Check sheet for the modelled part. Datum: model origin and axes. Units: mm. Give positions to 0.01 mm unless a question says otherwise; leave off trailing zeros. Write each loop counter-clockwise with the first axis right and the second up, starting at its lowest first coordinate (ties: lowest second). Pieces come first, ordered by that corner, then holes. Notation, with made-up numbers: M 18.5,55.5 L 29.5,55.5 A26 ccw 29.5,73.5 Z; hole C -8.75,37 d8. An arc over 180 degrees is marked long. Use CSV: the item, a comma, the result in double quotes. Start each with the question number.
1. Mould release check, pull along X, two halves, no side actions. Record for faces 1 (the face through (76.833, 5.164, 1.252)), 2 (the face through (6.67, 11.11, 1.25)), 3 (the face through (39, 5, 2.54)): +X half, -X half, draft (parallel to the pull), parting line (faces both ways), or undercut.
2. Cross-section at C-C, the plane y = 8.75. Enter the section's corners in (x, z).
3. Cross-section at B-B, the plane z = 0.9. Enter the section's corners in (x, y) (3 decimals).
4. Cross-section at A-A, the plane y = 5.08. Enter the section's corners in (x, z) (3 decimals), and give its area (3 significant figures).
5. Cross-section at D-D, the plane y = 2. Enter the section's corners in (x, z).
6. Scan lines: line 1 (X direction, y = 5, z = 1.7); line 2 (Y direction, x = 74.93, z = 0.6) (3 decimals); line 3 (X direction, y = 6.75, z = 0.4). Record each from-to range of solid material in increasing order.
from build123d import *

# Parameters (mm, degrees)
SKETCH1_R           = 1.905
BOSS_EXTRUDE1_DEPTH = 2.54
FILLET7_R           = 5.08


with BuildPart() as part:
    # Sketch1 → Boss-Extrude1 (new body)
    with BuildSketch(Plane.XY):
        Polygon((5.08, 10.16), (6.35, 11.43), (40.005, 11.43), (40.005, -1.27), (6.35, -1.27), (5.08, 0), (0, 0), (0, 10.16), align=None)
        with Locations((5.08, 5.08)):
            Circle(SKETCH1_R, mode=Mode.SUBTRACT)
    extrude(amount=BOSS_EXTRUDE1_DEPTH)

    # Fillet7
    # the kernel refuses this fillet: 5.08 mm, written as the material it takes off along each edge
    with BuildSketch(Plane(origin=(6.35, -1.27, -5.225260413), x_dir=(1, 0, 0), z_dir=(0, 0, 1))) as fillet7_piece_1:
        with BuildLine():
            CenterArc((2.090104165, 5.08), FILLET7_R, 228.590377891, 41.409622109)
            Line((-1.27, 1.27), (-1.337202083, 1.1938))
            ThreePointArc((-1.337202083, 1.1938), (-0.706842049, 0.563157951), (-0.071842049, -0.071842049))
            Line((-0.071842049, -0.071842049), (0, -0.1016))
            Line((0, -0.1016), (2.090104165, -0.1016))
            Line((2.090104165, -0.1016), (2.090104165, 0))
        make_face()
    extrude(amount=12.990520825, mode=Mode.SUBTRACT)
    with BuildSketch(Plane(origin=(6.35, 11.43, -5.225260413), x_dir=(-0.7071067811865464, -0.7071067811865488, 0), z_dir=(0, 0, 1))) as fillet7_piece_2:
        with BuildLine():
            CenterArc((2.11417562, 5.070029277), FILLET7_R, 225, 41.409622109)
            Line((-1.477926828, 1.477926828), (-1.549768877, 1.40608478))
            Line((-1.549768877, 1.40608478), (-0.071842049, -0.071842049))
            Line((-0.071842049, -0.071842049), (0, -0.1016))
            ThreePointArc((0, -0.1016), (0.898025612, -0.1016), (1.789688736, -0.101400586))
            Line((1.789688736, -0.101400586), (1.796051224, 0))
        make_face()
    extrude(amount=12.990520825, mode=Mode.SUBTRACT)
    with BuildSketch(Plane(origin=(0, 0, -12.7), x_dir=(1, 0, 0), z_dir=(0, 0, 1)), Plane(origin=(0, 10.16, -12.7), x_dir=(0, -1, 0), z_dir=(0, 0, 1))) as fillet7_piece_3:
        with BuildLine():
            CenterArc((FILLET7_R, FILLET7_R), FILLET7_R, 180, 90)
            Line((0, FILLET7_R), (-FILLET7_R * 0.02, FILLET7_R))
            Line((-FILLET7_R * 0.02, FILLET7_R), (-FILLET7_R * 0.02, -FILLET7_R * 0.02))
            Line((-FILLET7_R * 0.02, -FILLET7_R * 0.02), (FILLET7_R, -FILLET7_R * 0.02))
            Line((FILLET7_R, -FILLET7_R * 0.02), (FILLET7_R, 0))
        make_face()
    extrude(amount=27.94, mode=Mode.SUBTRACT)

    # Mirror7: part across plane


with BuildPart() as part_1:
    add(part.part)
    add(part.part.mirror(Plane(origin=(40.005, -1.27, 2.54), x_dir=(0, 0, 1), z_dir=(-1, 0, 0))))


solid = part_1.part
Worked answers:
1,face 1,"undercut"
1,face 2,"-X half"
1,face 3,"draft"
2,outline,"M 1.57,0 L 78.44,0 L 78.44,2.54 L 1.57,2.54 Z"
3,outline,"M 5.08,0 A5.08 ccw 8.44,-1.27 L 71.57,-1.27 A5.08 ccw 74.93,0 A5.08 ccw 74.93,10.16 A5.08 ccw 71.57,11.43 L 8.44,11.43 A5.08 ccw 5.08,10.16 A5.08 ccw Z; hole C 5.08,5.08 d3.81; hole C 74.93,5.08 d3.81"
4,outline,"M 0,0 L 3.175,0 L 3.175,2.54 L 0,2.54 Z; M 6.985,0 L 73.025,0 L 73.025,2.54 L 6.985,2.54 Z; M 76.835,0 L 80.01,0 L 80.01,2.54 L 76.835,2.54 Z"
4,area,"184 mm^2"
5,outline,"M 1.04,0 L 78.97,0 L 78.97,2.54 L 1.04,2.54 Z"
6,line 1,"x = 0 to 3.18, 6.98 to 73.03, 76.83 to 80.01"
6,line 2,"y = 0 to 3.175, 6.985 to 10.16"
6,line 3,"x = 0.28 to 4.16, 6 to 74.01, 75.85 to 79.73"
